```python
from build123d import *

# Parameters (mm, degrees)
F1_DEPTH = 30


with BuildPart() as f1:
    # F0 (on Top) → F1 (new body)
    with BuildSketch(Plane.XY):
        with BuildLine():
            Line((8.036751, 47.808975), (-41.963249, 47.808975))
            ThreePointArc((-41.963249, 47.808975), (-57.904896, 45.774272), (-67.202643, 32.665953))
            Line((-67.202643, 32.665953), (-67.202643, -37.334047))
            Line((-67.202643, -37.334047), (-37.202643, -37.334047))
            Line((-37.202643, -37.334047), (-37.202643, -17.334047))
            ThreePointArc((-37.202643, -17.334047), (-27.202643, -7.334047), (-17.202643, -17.334047))
            Line((-17.202643, -17.334047), (-17.202643, -37.334047))
            Line((-17.202643, -37.334047), (42.797357, -37.334047))
            Line((42.797357, -37.334047), (42.797357, -17.334047))
            ThreePointArc((42.797357, -17.334047), (52.347088, -10.300972), (61.896819, -17.334047))
            Line((61.896819, -17.334047), (61.896819, -37.334047))
            Line((61.896819, -37.334047), (101.896819, -37.334047))
            Line((101.896819, -37.334047), (101.896819, 6.665953))
            Line((101.896819, 6.665953), (70.641249, 47.808975))
            Line((70.641249, 47.808975), (35.641249, 47.808975))
            Line((35.641249, 47.808975), (35.641249, 17.808975))
            ThreePointArc((35.641249, 17.808975), (21.839, 8.682468), (8.036751, 17.808975))
            Line((8.036751, 17.808975), (8.036751, 47.808975))
        make_face()
    extrude(amount=F1_DEPTH)


solid = f1.part
```
The listing builds one solid part. Answer for the finished solid, in the listing's coordinates (mm). A direction names the side the tool comes from. Round coordinates to 2 decimals unless told otherwise and drop trailing zeros. Loops run counter-clockwise (first coordinate to the right, second up) from the corner with the lowest first, then second, coordinate; pieces in that order, holes last. Notation, with made-up numbers: (4, 64.5) - (50, 64.5) arc R22 ccw to (50, 83.5) - close; hole circle Ø11 at (81, -9). An arc over 180 degrees is marked (long way). Use one line per item in the form item = value. Start each with the question number.
1. The part is cut by section A-A on z = 18. Determine the outline of the cut face in (x, y), then the cut area to 3 significant figures.
2. Consider line 1 (X direction, y = -12, z = 28.75); line 2 (Y direction, x = -8.5, z = 3.5); line 3 (X direction, y = 42.5, z = 20). Determine where each line is inside the solid, lowest interval first. Write a range as [from, to].
3. For a pull along X with two mould halves and no side action, classify faces 5 (the face through (101.897, -16, 15)), 6 (the face through (-67.203, -2, 15)), 7 (the face through (-17.203, -27, 15)), 8 (the face through (16, 6, 0)) as pulls with the +X half, pulls with the -X half, needs draft (parallel to the pull), parting line crosses it, or undercut.
4. The part is cut by section B-B on y = 38. Determine the outline of the cut face in (x, z), then the cut area to 3 significant figures.
5. Given pin 1 Ø12 at (x, z) = (57.5, 23) entering from +Y; pin 2 Ø15 at (y, z) = (35, 10.5) entering from -X; pin 3 Ø9 at (y, z) = (31, 8) entering from +X, each flat-ended and moving along its own axis, determine where each tip first touches the part or whether it passes through.
6. The part is cut by section C-C on y = 22.5. Determine the outline of the cut face in (x, z).
7. The part is cut by section D-D on x = 55. Determine the outline of the cut face in (y, z).
8. A tool of negligible diameter and unlimited length cuts with its end or side. For faces 1 (the face through (53, 47.809, 15)), 2 (the face through (82, -37.334, 15)), 3 (the face through (8.037, 33, 15)), 4 (the face through (-37.203, -27, 15)), from which of +Z, -Z, +X, -X, +Y, -Y can it reach the whole face along a straight path? Write none if from no direction.
Geometry check:
q1.outline = (-67.2, -37.33) - (-37.2, -37.33) - (-37.2, -17.33) arc R10 cw to (-17.2, -17.33) - (-17.2, -37.33) - (42.8, -37.33) - (42.8, -17.33) arc R10 cw to (61.9, -17.33) - (61.9, -37.33) - (101.9, -37.33) - (101.9, 6.67) - (70.64, 47.81) - (35.64, 47.81) - (35.64, 17.81) arc R15 cw to (8.04, 17.81) - (8.04, 47.81) - (-41.96, 47.81) arc R20 ccw to (-67.2, 32.67) - close
q1.area = 11,600 mm^2
q2.line_1 = [-67.2, -35.66], [-18.74, 46.77], [57.92, 101.9]
q2.line_2 = [-37.33, 47.81]
q2.line_3 = [-62.02, 8.04], [35.64, 74.67]
q3.face_5 = pulls with the +X half
q3.face_6 = pulls with the -X half
q3.face_7 = undercut
q3.face_8 = needs draft
q4.outline = (-65.28, 0) - (8.04, 0) - (8.04, 30) - (-65.28, 30) - close; (35.64, 0) - (78.09, 0) - (78.09, 30) - (35.64, 30) - close
q4.area = 3,470 mm^2
q5.pin_1 = 47.81
q5.pin_2 = -67.2
q5.pin_3 = 86.83
q6.outline = (-67.2, 0) - (8.04, 0) - (8.04, 30) - (-67.2, 30) - close; (35.64, 0) - (89.87, 0) - (89.87, 30) - (35.64, 30) - close
q7.outline = (-10.66, 0) - (47.81, 0) - (47.81, 30) - (-10.66, 30) - close
q8.face_1 = +Z, -Z, +X, +Y
q8.face_2 = +Z, -Z, +X, -X, -Y
q8.face_3 = +Z, -Z, +Y
q8.face_4 = +Z, -Z, -Y
